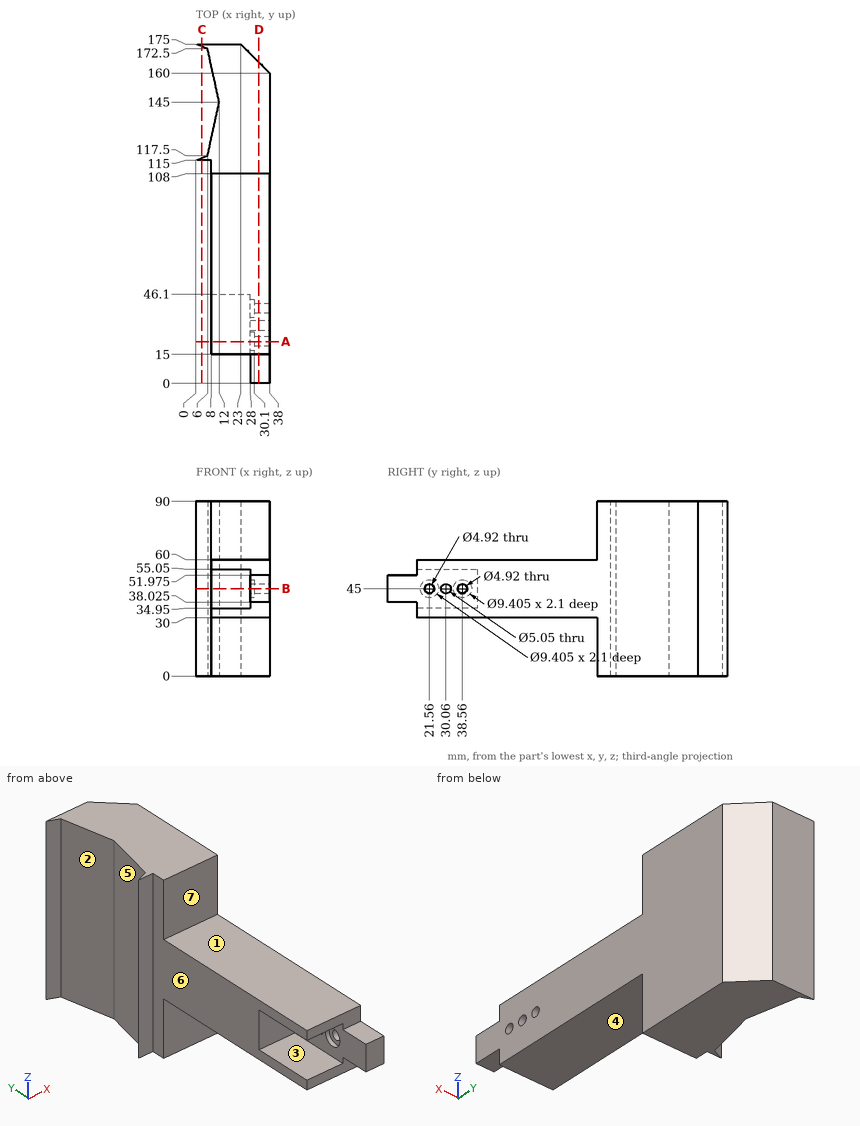
The drawing under review shows one solid part. Ordinate dimensions are in mm from its lowest x, y, z. A direction names the side the tool comes from. Round coordinates to 2 decimals unless told otherwise and drop trailing zeros. Order: outer loops, then holes, each group sorted by start corner. A loop starts at its lowest first (then second) coordinate and runs counter-clockwise, first axis right, second up. Notation, with made-up numbers: M 7,39 L 39,39 A22 ccw 39,69 Z; hole C 80,41 d1. An arc over 180 degrees is marked long. Answer as CSV lines item,"result". Start each with the question number.
1) Add section C-C (x = 3). Give the boundary of the cut face in (y, z).
2) Wall thickness on line 1 along Z through (x, y) = (23.5, 45.5); line 2 along Z through (x, y) = (34.5, 21.56); line 3 along Y through (x, z) = (28.5, 45) (1 decimal): over which ranges is each line inside the solid? List them lowest first. Write a range as [from, to].
3) The part is to be moulded in two halves that separate along Z. For the marked faces 1, 2 and 3, say which applies: +Z half, -Z half, draft (parallel to the pull), parting line (faces both ways), or undercut.
4) Tool access review of the marked faces 4, 5, 6 and 7: name each direction out of +Z, -Z, +X, -X, +Y, -Y from which nothing blocks a thin tool from reaching the whole face with its end or side.
5) Add section D-D (x = 32.5). Give the boundary of the cut face in (y, z) (3 decimals), then the cut area to 3 significant figures.
6) For pin 1 Ø16 at (x, y) = (17, 29.5) entering from -Z; pin 2 Ø16 at (x, y) = (13.5, 29) entering from +Z; pin 3 Ø4 at (x, z) = (16.5, 56) entering from -Y; pin 4 Ø6 at (y, z) = (89.5, 64.5) entering from +X, all flat-tipped, find the tip position at first contact; note any pin that passes through.
7) Add section B-B (z = 45). Give the number of separate pieces and of enclosed holes in the cut face, then the cut area to 3 significant figures.
8) Add section A-A (y = 21.56). Give the boundary of the cut face in (x, z).
Resolved:
1,outline,"M 115,0 L 116.25,0 L 116.25,90 L 115,90 Z; M 173.75,0 L 175,0 L 175,90 L 173.75,90 Z"
2,line 1,"[30, 34.95], [55.05, 60]"
2,line 2,"[30, 42.54], [47.46, 60]"
2,line 3,"[0, 16.9], [26.3, 27.5], [32.6, 33.9], [43.3, 169.5]"
3,face 1,"+Z half"
3,face 2,"draft"
3,face 3,"undercut"
4,face 4,"-Z, +X, -X, -Y"
4,face 5,"+Z, -Z, -X"
4,face 6,"+Z, -Z, -X, -Y"
4,face 7,"+Z, +X, -X, -Y"
5,outline,"M 0,38.025 L 15,38.025 L 15,30 L 108,30 L 108,0 L 165.5,0 L 165.5,90 L 108,90 L 108,60 L 15,60 L 15,51.975 L 0,51.975 Z; hole C 21.56,45 d4.92; hole C 30.06,45 d5.05; hole C 38.56,45 d4.92"
5,area,"8,120 mm^2"
6,pin 1,"z = 30"
6,pin 2,"z = 60"
6,pin 3,"y = 15"
6,pin 4,"through"
7,separate pieces,"4"
7,enclosed holes,"0"
7,area,"4,020 mm^2"
8,outline,"M 8,30 L 38,30 L 38,42.54 L 30.1,42.54 L 30.1,40.3 L 28,40.3 L 28,34.95 L 8,34.95 Z; M 8,55.05 L 28,55.05 L 28,49.7 L 30.1,49.7 L 30.1,47.46 L 38,47.46 L 38,60 L 8,60 Z"
